from build123d import *

# Parameters (mm, degrees)
BOSS_EXTRUDE1_DEPTH      = 10
BOSS_EXTRUDE1_DEPTH_BACK = 10
SKETCH1_R                = 6.5
SKETCH1_R_2              = 4.5
CUT_EXTRUDE2_DEPTH       = 6
CUT_EXTRUDE3_DEPTH       = 6
SKETCH4_R                = 6.5
SKETCH4_R_2              = 6.3
CUT_EXTRUDE4_DEPTH       = 23.011360703


with BuildPart() as part:
    # Sketch1 → Boss-Extrude1 (new, two sides: drawn at the far end of the back side and taken through both)
    with BuildSketch(Plane.XY.offset(-BOSS_EXTRUDE1_DEPTH_BACK)):
        Circle(SKETCH1_R)
        Circle(SKETCH1_R_2, mode=Mode.SUBTRACT)
    extrude(amount=BOSS_EXTRUDE1_DEPTH + BOSS_EXTRUDE1_DEPTH_BACK)

    # Sketch2 → Cut-Extrude2 (cut)
    with BuildSketch(Plane.XY.offset(10)):
        with BuildLine():
            Line((-6.230040483, 9.970148902), (0, 0))
            Line((0, 0), (0, 11.756584264))
            ThreePointArc((0, 11.756584264), (-3.2405538, 11.301154128), (-6.230040483, 9.970148902))
        make_face()
    extrude(amount=-CUT_EXTRUDE2_DEPTH, mode=Mode.SUBTRACT)

    # Sketch3 → Cut-Extrude3 (cut)
    with BuildSketch(Plane.XY.offset(-10)):
        with BuildLine():
            Line((-6.230040483, 9.970148902), (0, 0))
            Line((0, 0), (0, 11.756584264))
            ThreePointArc((0, 11.756584264), (-3.2405538, 11.301154128), (-6.230040483, 9.970148902))
        make_face()
    extrude(amount=CUT_EXTRUDE3_DEPTH, mode=Mode.SUBTRACT)

    # Sketch4 → Cut-Extrude4 (cut, through all)
    with BuildSketch(Plane(origin=(0, 0, -10), x_dir=(-1, 0, 0), z_dir=(0, 0, -1))):
        Circle(SKETCH4_R)
        with Locations(Location((0, 0, 0), (0, 0, 58))):
            Circle(SKETCH4_R_2, mode=Mode.SUBTRACT)
    extrude(amount=-CUT_EXTRUDE4_DEPTH, mode=Mode.SUBTRACT)


solid = part.part
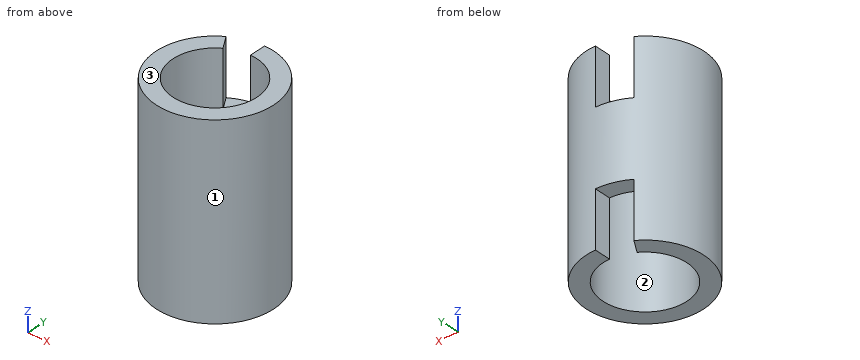
Read the model definition and answer for the solid it produces. Units are mm, in the model's axes. Face numbers are marked on the shaded views. Round coordinates to 2 decimals unless told otherwise and drop trailing zeros. Write each loop counter-clockwise with the first axis right and the second up, starting at its lowest first coordinate (ties: lowest second). Pieces come first, ordered by that corner, then holes. Notation, with made-up numbers: (12.5, 43.5) - (68.5, 43.5) arc R11 ccw to (68.5, 50.5) - close; hole circle Ø11 at (-19.75, 33). An arc over 180 degrees is marked (long way). One line per question, with ' | ' between items. Start each with the question number.
1. Section A-A (y = 0) is taken. Determine the outline of the cut face in (x, z), and give its area (3 significant figures).
2. Section C-C (z = 1.75) is taken. Determine the outline of the cut face in (x, y).
3. Find the intervals of material crossed by probe 1 along Y at (x, z) = (0, -2.5); probe 2 along Y at (x, z) = (-3.75, -1.5), in increasing order. Write a range as [from, to].
4. Section D-D (y = 5.75) is taken. Determine the outline of the cut face in (x, z).
5. For a pull along X with two mould halves and no side action, classify the marked faces 1, 2 and 3 as +X half, -X half, draft (parallel to the pull), parting line (faces both ways), or undercut.
6. Each of these flat-tipped pins is pushed along its axis until it touches: pin 1 (4 mm diameter, centred on x = -4, z = -6, fed in from -Y); pin 2 (1.5 mm diameter, centred on x = -1.5, y = 1, fed in from +Z); pin 3 (0.7 mm diameter, centred on x = -2, y = 5.5, fed in from -Z); pin 4 (1.5 mm diameter, centred on x = 2.5, z = 1, fed in from -Y). Where does it stop, or does it pass through?
7. Section B-B (x = -1.5) is taken. Determine the outline of the cut face in (y, z).
Filled in:
1) outline: (-6.3, -10) - (-4.5, -10) - (-4.5, 10) - (-6.3, 10) - close; (4.5, -10) - (6.3, -10) - (6.3, 10) - (4.5, 10) - close | area: 72.0 mm²
2) outline: circle Ø12.6 at (0, 0); hole circle Ø9 at (0, 0)
3) probe 1: [-6.3, -4.5], [4.5, 6.3] | probe 2: [-5.06, -2.49], [2.49, 5.06]
4) outline: (-2.57, -4) - (0, -4) - (0, -10) - (2.57, -10) - (2.57, 10) - (0, 10) - (0, 4) - (-2.57, 4) - close
5) face 1: parting line | face 2: undercut | face 3: draft
6) pin 1: y = -5.97 | pin 2: through | pin 3: z = -4 | pin 4: y = -6.05
7) outline: (-6.12, -10) - (-4.24, -10) - (-4.24, 10) - (-6.12, 10) - close; (4.24, -4) - (6.12, -4) - (6.12, 4) - (4.24, 4) - close
